Geometry check sheet. Reference: drawing and pictorial views, mm from the part's lowest x, y, z. A direction names the side the tool comes from. Round coordinates to 2 decimals unless told otherwise and drop trailing zeros. Order: outer loops, then holes, each group sorted by start corner. A loop starts at its lowest first (then second) coordinate and runs counter-clockwise, first axis right, second up.
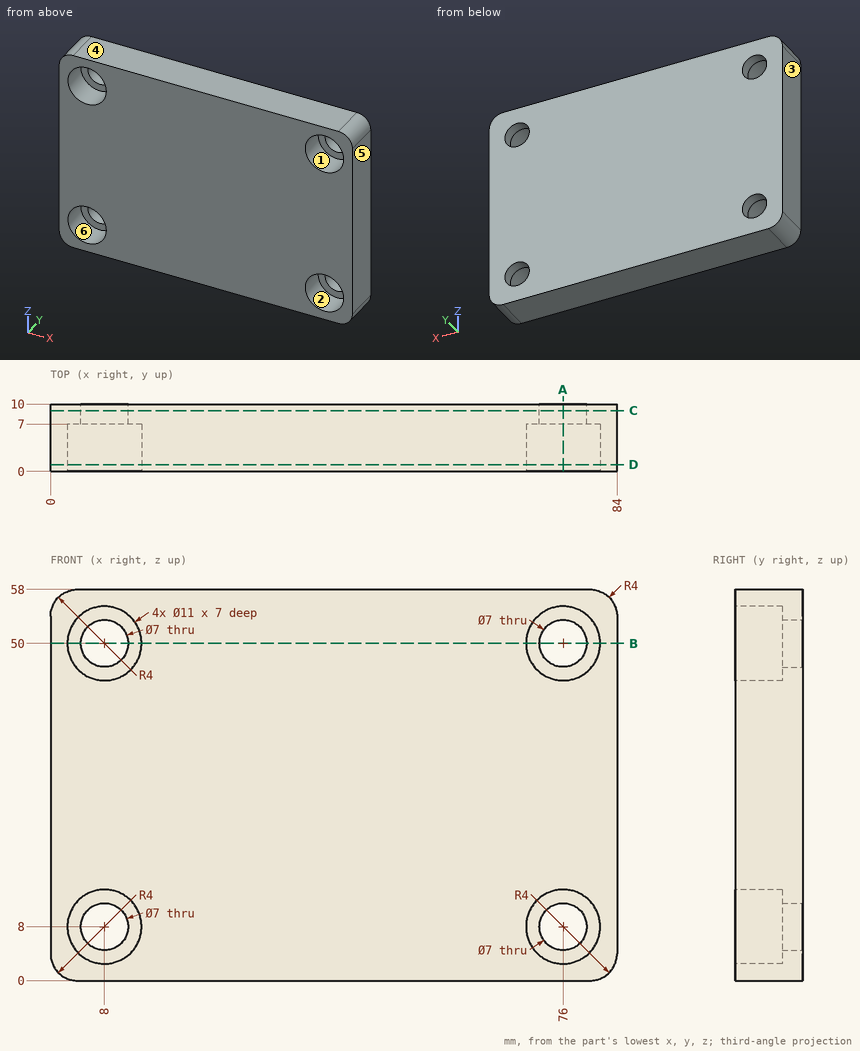
1) Sectioned sample at A-A on x = 76. Record the cut outline in (y, z).
2) Go/stop test with a flat-tipped pin: pin 1 Ø10 at (x, z) = (8, 8) entering from -Y. Record where the tip stops, or that it passes through.
3) Draft check along Z on the marked faces 1, 2, 3 and 4. Enter one of: released by +Z, released by -Z, zero draft, split by the parting line, or undercut.
4) Sectioned sample at C-C on y = 9. Record the cut outline in (x, z), then the cut area to 3 significant figures.
5) Scan lines: probe 1 along Z at (x, y) = (76, 8.1); probe 2 along Z at (x, y) = (76, 2); probe 3 along X at (y, z) = (8.5, 51.5). Record each from-to range of solid material in increasing order.
6) Sectioned sample at B-B on z = 50. Record the cut outline in (x, y).
7) Tool access check on the marked faces 5 and 6. Record the directions out of +Z, -Z, +X, -X, +Y, -Y that give a thin tool (end or side, any length) a straight path to the whole face; none if there is none.
8) Sectioned sample at D-D on y = 1. Record the cut outline in (x, z).
Returned:
1. outline: (0, 0) - (10, 0) - (10, 4.5) - (7, 4.5) - (7, 2.5) - (0, 2.5) - close; (0, 13.5) - (7, 13.5) - (7, 11.5) - (10, 11.5) - (10, 46.5) - (7, 46.5) - (7, 44.5) - (0, 44.5) - close; (0, 55.5) - (7, 55.5) - (7, 53.5) - (10, 53.5) - (10, 58) - (0, 58) - close
2. pin 1: stops at y = 7
3. face 1: undercut
3. face 2: undercut
3. face 3: zero draft
3. face 4: released by +Z
4. outline: (0, 4) arc R4 ccw to (4, 0) - (80, 0) arc R4 ccw to (84, 4) - (84, 54) arc R4 ccw to (80, 58) - (4, 58) arc R4 ccw to (0, 54) - close; hole circle Ø7 at (8, 8); hole circle Ø7 at (8, 50); hole circle Ø7 at (76, 8); hole circle Ø7 at (76, 50)
4. area: 4,700 mm2
5. probe 1: z = 0 to 4.5, 11.5 to 46.5, 53.5 to 58
5. probe 2: z = 0 to 2.5, 13.5 to 44.5, 55.5 to 58
5. probe 3: x = 0 to 4.84, 11.16 to 72.84, 79.16 to 84
6. outline: (0, 0) - (2.5, 0) - (2.5, 7) - (4.5, 7) - (4.5, 10) - (0, 10) - close; (11.5, 7) - (13.5, 7) - (13.5, 0) - (70.5, 0) - (70.5, 7) - (72.5, 7) - (72.5, 10) - (11.5, 10) - close; (79.5, 7) - (81.5, 7) - (81.5, 0) - (84, 0) - (84, 10) - (79.5, 10) - close
7. face 5: +Z, -Z, +X, +Y, -Y
7. face 6: -Y
8. outline: (0, 4) arc R4 ccw to (4, 0) - (80, 0) arc R4 ccw to (84, 4) - (84, 54) arc R4 ccw to (80, 58) - (4, 58) arc R4 ccw to (0, 54) - close; hole circle Ø11 at (8, 8); hole circle Ø11 at (8, 50); hole circle Ø11 at (76, 8); hole circle Ø11 at (76, 50)
